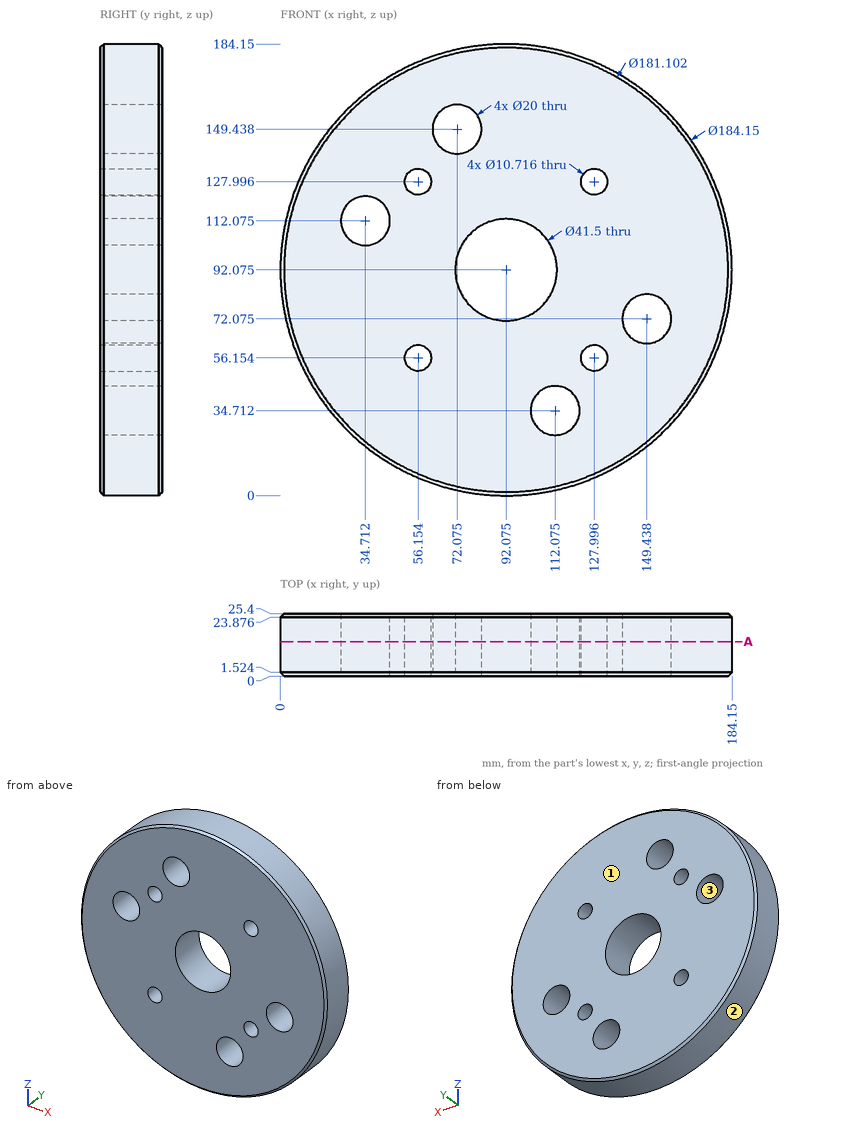
For this review, use the dimensioned drawing (mm, ordinates from the lowest corner) and the shaded views. Give positions to 0.01 mm unless a question says otherwise; leave off trailing zeros. Write item = value, one per line. Start each with the question number.
(1) Take a section at A-A (y = 14). State how many separate pieces and enclosed holes the cut face has, plus the area to 3 significant figures.
(2) For L1, parallel to X at y = 21, z = 60 (1 decimal); L2, parallel to Z at x = 105, y = 7.5 (1 decimal); L3, parallel to Z at x = 92.5, y = 21.25, list the stretches that pass through material, from the lowest coordinate up. Write a range as from..to.
(3) For pin 1 Ø10 at (x, y) = (53.5, 8) entering from -Z; pin 2 Ø1.5 at (x, y) = (164.5, 11) entering from +Z; pin 3 Ø10 at (y, z) = (15.5, 34.5) entering from -X (1 decimal); pin 4 Ø6.5 at (x, z) = (128, 56.15) entering from -Y, all flat-tipped, find the tip position at first contact; note any pin that passes through.
(4) Draft analysis for pull direction Z (two halves, no side actions). For the marked faces 1, 2 and 3, state which applies: +Z half, -Z half, draft (parallel to the pull), parting line (faces both ways), or undercut.
Returned:
q1.separate_pieces = 1
q1.enclosed_holes = 9
q1.area = 23,700 mm²
q2.L1 = 5.8..52.4, 59.9..124.3, 131.7..178.4
q2.L2 = 0.9..27.6, 41.8..75.8, 108.3..183.2
q2.L3 = 0..71.33, 112.82..184.15
q3.pin_1 = 6.34
q3.pin_2 = 149.87
q3.pin_3 = 16.5
q3.pin_4 = through
q4.face_1 = draft
q4.face_2 = parting line
q4.face_3 = undercut
